Could you check a few things on this model? Use its own coordinates, in mm. A direction names the side the tool comes from. Round coordinates to 2 decimals unless told otherwise and drop trailing zeros. Write each loop counter-clockwise with the first axis right and the second up, starting at its lowest first coordinate (ties: lowest second). Pieces come first, ordered by that corner, then holes. Notation, with made-up numbers: M 60.5,60.5 L 93.5,60.5 A21 cw 93.5,70.5 Z; hole C -29.5,24 d4. An arc over 180 degrees is marked long. One line per question, with ' | ' between items. Start each with the question number.
```python
from build123d import *

# Parameters (mm, degrees)
F0_W     = 152.4
F0_H     = 17.78
F0_W_2   = 17.78
F0_H_2   = 152.4
F1_DEPTH = 19.05


# Not quite as in the source:
# - a feature names something its author has since deleted; it is built from what else it names


with BuildPart() as f1:
    # F0 (on Right) → F1 (new body)
    with BuildSketch(Plane.YZ):
        with Locations((0, 8.89)):
            Rectangle(F0_W, F0_H)
        Polygon((-76.2, 0), (-228.6, 0), (-228.6, -336.55), (-76.2, -336.55), (76.2, -336.55), (228.6, -336.55), (228.6, -228.6), (228.6, -76.2), (228.6, 0), (76.2, 0), align=None)
        with Locations((237.49, -152.4)):
            Rectangle(F0_W_2, F0_H_2)
        with Locations((0, -345.44)):
            Rectangle(F0_W, F0_H)
    extrude(amount=F1_DEPTH)


solid = f1.part
```
1. I need wall thicknesses on line 1 along Y through (x, z) = (6.5, -32.5); line 2 along Z through (x, y) = (5, -131.5). Which ranges of each line are inside material? Lowest first, please. Write a range as from..to.
2. Suppose I cut it at C-C (y = 186.5). Write out the boundary of the cut face in (x, z), and give its area (3 significant figures).
3. Suppose I cut it at A-A (x = 3.25). Write out the boundary of the cut face in (y, z).
4. Which directions (+Z, -Z, +X, -X, +Y, -Y) give clear straight access to the entire face, cutting with the end or side of a thin tool? Please do faces 1 (the face through (9, -153, -336.55)), 2 (the face through (9, 76.2, -346)), 3 (the face through (9, -151, 0)).
5. I'm going to push flat-ended pins straight in: P1, Ø5.5, axis at x = 6.5, y = 183, coming from the +Z side; P2, Ø5.5, axis at x = 13, z = -40, coming from the +Y side; P3, Ø5.5, axis at x = 8, z = 5, coming from the -Y side. Where does each tip first touch, or does it pass through?
6. Suppose I cut it at B-B (z = -260). Write out the boundary of the cut face in (x, y), and give its area (3 significant figures).
Computed:
1) line 1: y = -228.6..228.6 | line 2: z = -336.55..0
2) outline: M 0,-336.55 L 19.05,-336.55 L 19.05,0 L 0,0 Z | area: 6,410 mm²
3) outline: M -228.6,-336.55 L -76.2,-336.55 L -76.2,-354.33 L 76.2,-354.33 L 76.2,-336.55 L 228.6,-336.55 L 228.6,-228.6 L 246.38,-228.6 L 246.38,-76.2 L 228.6,-76.2 L 228.6,0 L 76.2,0 L 76.2,17.78 L -76.2,17.78 L -76.2,0 L -228.6,0 Z
4) face 1: -Z, +X, -X, -Y | face 2: -Z, +X, -X, +Y | face 3: +Z, +X, -X, -Y
5) P1: stops at z = 0 | P2: stops at y = 228.6 | P3: stops at y = -76.2
6) outline: M 0,-228.6 L 19.05,-228.6 L 19.05,228.6 L 0,228.6 Z | area: 8,710 mm²
